Autodesk Inventor part; units mm, degrees
ref_plane "YZ Plane" through (0, 0, 0) normal (1, 0, 0) x (0, 1, 0)
ref_plane "XZ Plane" through (0, 0, 0) normal (0, 1, 0) x (-1, 0, 0)
ref_plane "XY Plane" through (0, 0, 0) normal (0, 0, 1) x (1, 0, 0)
sketch "Sketch1" plane through (0, 0, 0) normal (0, 1, 0) x (-1, 0, 0)
  line L0 (0, 0) -> (0, -85.5)
  line L1 (0, -85.5) -> (127.8, -85.5)
  line L2 (127.8, -85.5) -> (127.8, 0)
  line L3 (127.8, 0) -> (0, 0)
  dimension "d0" = 85.5
  dimension "d1" = 127.8
extrude "Extrusion2" add sketch "Sketch1" along normal blind 7
sketch "Sketch3" plane through (0, 7, 0) normal (0, 1, 0) x (1, 0, 0)
  point P0 (0, 0)
sketch "Sketch4" plane through (0, 7, 0) normal (0, 1, 0) x (1, 0, 0)
  arc A0 (-87.0052, 57.9703) -> (-87.3264, 30.9885) centre (-90.5182, 44.5193) ccw
  arc A1 (-88.9325, 52.5097) -> (-88.9325, 35.4855) centre (-89.7687, 43.9976) ccw
  line L0 (-88.9325, 52.5097) -> (-87.0052, 57.9703)
  line L1 (-88.9325, 35.4855) -> (-87.3264, 30.9885)
  arc A2 (-73.8153, 53.315) -> (-74.072, 35.7223) centre (-72.2893, 44.4945) ccw
  arc A3 (-70.5066, 35.7223) -> (-70.7634, 53.315) centre (-72.2893, 44.4945) ccw
  arc A4 (-70.7634, 30.9885) -> (-70.7634, 57.9703) centre (-71.8849, 44.4794) ccw
  line L2 (-70.7634, 57.9703) -> (-70.7634, 53.315)
  line L3 (-70.5066, 35.7223) -> (-70.7634, 30.9885)
  line L4 (-74.072, 35.7223) -> (-74.072, 30.7346)
  line L5 (-73.8153, 57.9703) -> (-73.8153, 53.315)
  arc A5 (-73.8153, 57.9703) -> (-74.072, 30.7346) centre (-73.6823, 44.35) ccw
  line L6 (-54.7714, 57.9703) -> (-54.7714, 30.7346)
  line L7 (-54.7714, 30.7346) -> (-50.7714, 30.7346)
  line L8 (-50.7714, 30.7346) -> (-50.7714, 57.9703)
  line L9 (-50.7714, 57.9703) -> (-54.7714, 57.9703)
  line L10 (-43.1656, 30.7346) -> (-49.5383, 44.3525)
  arc A6 (-49.5383, 44.3525) -> (-49.5383, 55.6427) centre (-48.8397, 49.9976) ccw
  line L11 (-43.1656, 30.7346) -> (-39.7325, 32.3411)
  line L12 (-39.7325, 32.3411) -> (-44.3475, 42.2031)
  arc A7 (-44.3475, 42.2031) -> (-49.5383, 57.9703) centre (-47.7714, 49.814) ccw
  line L13 (-49.5383, 57.9703) -> (-49.5383, 55.6427)
  line L14 (-36.7714, 58.3504) -> (-36.7714, 30.7346)
  line L15 (-36.7714, 30.7346) -> (-22.7714, 30.7346)
  line L16 (-22.7714, 30.7346) -> (-22.7714, 35.5125)
  line L17 (-22.7714, 35.5125) -> (-32.7714, 35.5125)
  line L18 (-32.7714, 35.5125) -> (-32.7714, 43.7637)
  line L19 (-32.7714, 43.7637) -> (-24.9696, 43.7637)
  line L20 (-24.9696, 43.7637) -> (-24.9696, 46.7637)
  line L21 (-24.9696, 46.7637) -> (-32.7714, 46.7637)
  line L22 (-32.7714, 46.7637) -> (-32.7714, 54.7637)
  line L23 (-32.7714, 54.7637) -> (-22.7714, 54.7637)
  line L24 (-22.7714, 54.7637) -> (-22.7714, 58.3504)
  line L25 (-22.7714, 58.3504) -> (-36.7714, 58.3504)
  line L26 (-127.8, 85.5) -> (-127.8, 0)
  line L27 (0, 85.5) -> (-127.8, 85.5)
  point P0 (0, 0)
extrude "Extrusion3" cut sketch "Sketch4" against normal through all
sketch "Sketch5" plane through (0, 7, 0) normal (0, 1, 0) x (1, 0, 0)
  line L0 (-127.8, 0) -> (0, 0)
  line L1 (-127.8, 0) -> (0, 0)
  line L2 (0, 0) -> (0, 85.5)
  line L3 (0, 0) -> (0, 85.5)
  line L4 (0, 85.5) -> (-127.8, 85.5)
  line L5 (0, 85.5) -> (-127.8, 85.5)
  line L6 (-127.8, 85.5) -> (-127.8, 0)
  line L7 (-122.8, 80.5) -> (-5, 80.5)
  line L8 (-5, 80.5) -> (-5, 4.1226)
  line L9 (-5, 4.1226) -> (-122.8, 4.1226)
  line L10 (-122.8, 4.1226) -> (-122.8, 80.5)
  line L11 (-127.8, 85.5) -> (-127.8, 0)
  dimension "d44" = 5
  dimension "d45" = 5
  dimension "d46" = 5
extrude "Extrusion4" add sketch "Sketch5" along normal blind 10
sketch "Sketch9" plane through (0, 17, 0) normal (0, 1, 0) x (1, 0, 0)
  line L0 (-127.8, 85.5) -> (-127.8, 0)
  line L1 (-127.8, 0) -> (-127.8, 85.5)
  line L2 (-127.8, 85.5) -> (0, 85.5)
  line L3 (0, 85.5) -> (0, 0)
  line L4 (0, 0) -> (-127.8, 0)
  line L5 (-122.8, 4.1226) -> (-5, 4.1226)
  line L6 (-5, 80.5) -> (-122.8, 80.5)
  line L7 (-122.8, 4.1226) -> (-122.8, 80.5)
  line L8 (-122.8, 80.5) -> (-5, 80.5)
  line L9 (-5, 80.5) -> (-5, 4.1226)
  line L10 (-5, 4.1226) -> (-122.8, 4.1226)
  point P0 (0, 0)
ref_plane "Work Plane4" through (-63.9, 0, 0) normal (1, 0, 0) x (0, 0, -1)
sketch "Sketch21" plane through (-63.9, 0, 0) normal (1, 0, 0) x (0, 0, -1)
  line L0 (0, 0) -> (0, 17)
  line L1 (0, 7.0438) -> (0, 25.0438)
  line L2 (0, 25.0438) -> (-8, 25.0438)
  line L3 (-8, 25.0438) -> (0, 7.0438)
  line L4 (85.5, 0) -> (85.5, 17)
  line L5 (85.5, 7.0438) -> (85.5, 25.0438)
  line L6 (85.5, 25.0438) -> (93.5, 25.0438)
  line L7 (93.5, 25.0438) -> (85.5, 7.0438)
  dimension "d99" = 18
  dimension "d100" = 8
  dimension "d101" = 18
  dimension "d102" = 8
extrude "Extrusion7" add sketch "Sketch21" along normal mid plane 140
ref_plane "Work Plane5" through (-127.8, 0, -42.7) normal (0, 0, 1) x (1, 0, 0)
sketch "Sketch22" plane through (-127.8, 0, -42.7) normal (0, 0, 1) x (1, 0, 0)
  line L0 (127.8, 7.0438) -> (133.9, 7.0438)
  line L1 (127.8, 7.0438) -> (127.8, 25.0438)
  line L2 (133.9, 25.0438) -> (-6.1, 25.0438)
  line L3 (127.8, 25.0438) -> (135.8, 25.0438)
  line L4 (135.8, 25.0438) -> (127.8, 7.0438)
  line L5 (0, 0) -> (0, 7.0438)
  line L6 (0, 7.0438) -> (0, 25.0438)
  line L7 (0, 25.0438) -> (-8, 25.0438)
  line L8 (-6.1, 7.0438) -> (0, 7.0438)
  line L9 (-8, 25.0438) -> (0, 7.0438)
  point P0 (127.8, 0)
  dimension "d106" = 8
  dimension "d107" = 8
extrude "Extrusion8" add sketch "Sketch22" along normal mid plane 86
sketch "Sketch24" plane through (-127.8, 0, 0) normal (0, 0, 1) x (1, 0, 0)
  line L0 (-6.1, 7.0438) -> (-6.1, 25.0438)
  line L1 (0, 7.0438) -> (127.8, 7.0438)
  line L2 (-6.1, 20.9849) -> (0, 7.0438)
  line L3 (0, 7.0438) -> (-6.1, 7.0438)
  line L4 (-6.1, 7.0438) -> (-6.1, 20.9849)
  line L5 (127.8, 7.0438) -> (133.9, 7.0438)
  line L6 (133.9, 7.0438) -> (133.9, 20.7688)
  line L7 (127.8, 7.0438) -> (133.9, 20.7688)
  line L8 (133.9, 20.7688) -> (133.9, 7.0438)
  line L9 (133.9, 7.0438) -> (127.8, 7.0438)
  point P0 (127.8, 0)
extrude "Extrusion9" cut sketch "Sketch24" along normal blind 86
sketch "Sketch25" plane through (0, 0, -85.5) normal (0, 0, -1) x (-1, 0, 0)
  line L0 (-6.1, 20.7688) -> (0, 7.0438)
  line L1 (0, 7.0438) -> (-6.1, 20.7688)
  line L2 (-6.1, 20.7688) -> (-6.1, 7.0438)
  line L3 (-6.1, 7.0438) -> (0, 7.0438)
  line L4 (127.8, 7.0438) -> (133.9, 20.7688)
  line L5 (127.8, 7.0438) -> (133.9, 20.7688)
  line L6 (133.9, 7.0438) -> (133.9, 20.7688)
  line L7 (133.9, 20.7688) -> (133.9, 7.0438)
  line L8 (127.8, 7.0438) -> (0, 7.0438)
  line L9 (133.9, 7.0438) -> (127.8, 7.0438)
  point P0 (0, 0)
extrude "Extrusion10" cut sketch "Sketch25" along normal blind 86
properties part number "Rack holder Kinpen"
Geometry: final body of the model. Coordinates: model frame, mm. A direction names the side the tool comes from. Round coordinates to 2 decimals unless told otherwise and drop trailing zeros. Loops run counter-clockwise (first coordinate to the right, second up) from the corner with the lowest first, then second, coordinate; pieces in that order, holes last.
Item 1: Section D-D, the plane x = -8. Output: boundary loops of the cut face in (y, z), plus the area to 3 significant figures.
Checked values:
outline: (0, -85.5) - (7.04, -85.5) - (25.04, -93.5) - (25.04, -85.5) - (17, -85.5) - (17, -80.5) - (7, -80.5) - (7, -4.12) - (17, -4.12) - (17, 0) - (25.04, 0) - (25.04, 8) - (7.04, 0) - (0, 0) - close
area: 834 mm2
Item 2: Line query: L1, parallel to Z at x = -25.5, y = 3.75; L2, parallel to X at y = 7.5, z = -69; L3, parallel to Y at x = -65, z = -44.5. Output: solid intervals per line, ascending.
Checked values:
L1: z = -85.5 to -58.35, -54.76 to -46.76, -43.76 to -35.51, -30.73 to 0
L2: x = -128 to -122.8, -5 to 0.2
L3: y = 0 to 7
Item 3: Reachability of faces 4 (the flat face through (-65, 21, -85.5)), 5 (the flat face through (-41.47, 3.55, -31.53)), 6 (the flat face through (-133.9, 23, -89)) from +Z, -Z, +X, -X, +Y, -Y: full face, straight path, thin tool, end or side. Return the list, or none.
Checked values:
face 4: +Y
face 5: +Y, -Y
face 6: -Z, -X, +Y, -Y
Item 4: Mould query, pull axis X, two halves, no side actions, for faces 1 (the cylindrical face through (-81.236, 3.549, -44.799)), 2 (the flat face through (-63, 0, -33)), 3 (the flat face through (-131.856, 16.17, -46.293)). Classes: released by +X, released by -X, zero draft, split by the parting line, or undercut.
Checked values:
face 1: undercut
face 2: zero draft
face 3: released by -X
Item 5: Section C-C, the plane z = -12.5. Output: boundary loops of the cut face in (x, y).
Checked values:
outline: (-135.8, 25.04) - (-127.8, 7.04) - (-127.8, 0) - (0, 0) - (0, 7.04) - (8, 25.04) - (0, 25.04) - (0, 17) - (-5, 17) - (-5, 7) - (-122.8, 7) - (-122.8, 17) - (-127.8, 17) - (-127.8, 25.04) - close
Item 6: Section A-A, the plane x = -79. Output: boundary loops of the cut face in (y, z).
Checked values:
outline: (0, -85.5) - (7.04, -85.5) - (25.04, -93.5) - (25.04, -85.5) - (17, -85.5) - (17, -80.5) - (7, -80.5) - (7, -56.89) - (0, -56.89) - close; (0, -50.42) - (7, -50.42) - (7, -38.57) - (0, -38.57) - close; (0, -31.81) - (7, -31.81) - (7, -4.12) - (17, -4.12) - (17, 0) - (25.04, 0) - (25.04, 8) - (7.04, 0) - (0, 0) - close
Item 7: Contact query for flat-ended pins moving along their axis: P1, Ø12, axis at x = -39, z = -36, coming from the -Y side; P2, Ø12, axis at x = -113, z = -40.5, coming from the +Y side; P3, Ø7.5, axis at x = -28.5, y = 4, coming from the +Z side; P4, Ø3.5, axis at y = 22.5, z = 3.5, coming from the +X side. Output: stop coordinate, or through.
Checked values:
P1: stops at y = 0
P2: stops at y = 7
P3: stops at z = 0.31
P4: stops at x = 6.1
